Work out the finished part from the listing and answer in its coordinate system (mm). A direction names the side the tool comes from. Coordinates: 2 decimals unless noted, no trailing zeros. Order: outer loops, then holes, each group sorted by start corner. A loop starts at its lowest first (then second) coordinate and runs counter-clockwise, first axis right, second up. Notation, with made-up numbers: M -13,-40 L 10,-40 A21 cw 10,-18 Z; hole C -31.5,36 d6. An arc over 180 degrees is marked long. Use a Markdown table: item, result.
from build123d import *

# Parameters (mm, degrees)
SKETCH3_R        = 1.1303
SHAFT_DEPTH      = 12.7
TIP_SIZE         = 0.254
PHILLIPS_START   = 0.254
PHILLIPS_DEPTH   = 14.041159246
PHILLIPSFILLET_R = 0.127


with BuildPart() as part:
    # Sketch2 → Head (revolve)
    with BuildSketch(Plane(origin=(0, 0, 0), x_dir=(0, 0, -1), z_dir=(1, 0, 0))):
        with BuildLine():
            Line((0, 0), (2.7813, 0))
            ThreePointArc((2.7813, 0), (1.72225533, 1.469884796), (0, 2.032))
            Line((0, 2.032), (0, 0))
        make_face()
    revolve(axis=Axis((0, 0.415157056, 0), (0, -1, 0)))

    # Sketch3 → Shaft (add)
    with BuildSketch(Plane.XZ):
        with Locations(Location((0, 0, 0), (0, 0, 90))):
            Circle(SKETCH3_R)
    extrude(amount=SHAFT_DEPTH)

    # Tip
    tip_edges = [part.edges().sort_by_distance(p)[0] for p in [
        (0, -12.7, -1.1303),
    ]]
    chamfer(tip_edges, length=TIP_SIZE)

    # Sketch4 → Phillips (cut, through all)
    with BuildSketch(Plane(origin=(0, 0, 0), x_dir=(1, 0, 0), z_dir=(0, 1, 0)).offset(PHILLIPS_START)):
        Polygon((-0.4064, 0.4064), (-0.4064, 2.7813), (0.4064, 2.7813), (0.4064, 0.4064), (2.7813, 0.4064), (2.7813, -0.4064), (0.4064, -0.4064), (0.4064, -2.7813), (-0.4064, -2.7813), (-0.4064, -0.4064), (-2.7813, -0.4064), (-2.7813, 0.4064), align=None)
    extrude(amount=PHILLIPS_DEPTH, mode=Mode.SUBTRACT)

    # PhillipsFillet
    phillipsfillet_edges = [part.edges().sort_by_distance(p)[0] for p in [
        (0.4064, 1.114434201, -0.4064),
        (-0.4064, 1.114434201, -0.4064),
        (-0.4064, 1.114434201, 0.4064),
        (0.4064, 1.114434201, 0.4064),
    ]]
    fillet(phillipsfillet_edges, radius=PHILLIPSFILLET_R)


solid = part.part
1. Section B-B on x = 0 is taken. Determine the outline of the cut face in (y, z), then the cut area to 3 significant figures.
Answers below:
| item | result |
|---|---|
| outline | M -12.7,-0.88 L -12.45,-1.13 L 0,-1.13 L 0,-2.78 A2.92 ccw 0.25,-2.69 L 0.25,2.69 A2.92 ccw 0,2.78 L 0,1.13 L -12.45,1.13 L -12.7,0.88 Z |
| area | 30.0 mm² |
2. Section D-D on x = -1.85 is taken. Determine the outline of the cut face in (y, z), then the cut area to 3 significant figures.
Answers below:
| item | result |
|---|---|
| outline | M 0,-2.08 A2.26 ccw 1.33,-0.41 L 0.25,-0.41 L 0.25,0.41 L 1.33,0.41 A2.26 ccw 0,2.08 Z |
| area | 3.21 mm² |
3. For a pull along Z with two mould halves and no side action, classify faces 6 (the face through (-0.406, 1, -1)), 7 (the face through (-0.34, -6.14, 1.08)), 8 (the face through (1, 1, 0.406)) as +Z half, -Z half, draft (parallel to the pull), parting line (faces both ways), or undercut.
Answers below:
| item | result |
|---|---|
| face 6 | draft |
| face 7 | parting line |
| face 8 | undercut |
4. Section A-A on z = 0 is taken. Determine the outline of the cut face in (x, y), then the cut area to 3 significant figures.
Answers below:
| item | result |
|---|---|
| outline | M -2.78,0 L -1.13,0 L -1.13,-12.45 L -0.88,-12.7 L 0.88,-12.7 L 1.13,-12.45 L 1.13,0 L 2.78,0 A2.92 ccw 2.69,0.25 L -2.69,0.25 A2.92 ccw Z |
| area | 30.0 mm² |
5. Section C-C on y = -4.25 is taken. Determine the outline of the cut face in (x, z), then the cut area to 3 significant figures.
Answers below:
| item | result |
|---|---|
| outline | C 0,0 d2.26 |
| area | 4.01 mm² |
6. Flat-ended cylindrical pins translate along their axes: P1, Ø1.4, axis at y = 1, z = 1.5, coming from the +X side; P2, Ø0.5, axis at y = 1.5, z = 1.5, coming from the -X side; P3, Ø2, axis at x = -1.5, y = -8, coming from the +Z side. Find the tip coordinate at first contact, or state that the pin passes through.
Answers below:
| item | result |
|---|---|
| P1 | x = 2.37 |
| P2 | x = -1.39 |
| P3 | z = 1.01 |
7. Find the intervals of material crossed by probe 1 along X at (y, z) = (1.25, -1.05); probe 2 along Y at (x, z) = (-0.35, 0.65); probe 3 along Y at (x, z) = (2.2, 0.1), in increasing order.
Answers below:
| item | result |
|---|---|
| probe 1 | -1.69 to -0.41, 0.41 to 1.69 |
| probe 2 | -12.7 to 0.25 |
| probe 3 | 0 to 0.25 |
8. For faces 1 (the face through (1, 1, -0.406)), 2 (the face through (0.406, 1, 1)), 3 (the face through (-1, 0, 1)), 4 (the face through (0, 0.254, 0)), 5 (the face through (0, -12.7, 0)), determine the directions among +Z, -Z, +X, -X, +Y, -Y from which every point of the face is accessible in a straight line to the end or side of a thin tool.
Answers below:
| item | result |
|---|---|
| face 1 | +X, -X, +Y |
| face 2 | +Z, -Z, +Y |
| face 3 | -Y |
| face 4 | +Y |
| face 5 | +Z, -Z, +X, -X, -Y |
